Autodesk Inventor part; units mm, degrees
ref_plane "YZ Plane" through (0, 0, 0) normal (1, 0, 0) x (0, 1, 0)
ref_plane "XZ Plane" through (0, 0, 0) normal (0, 1, 0) x (-1, 0, 0)
ref_plane "XY Plane" through (0, 0, 0) normal (0, 0, 1) x (1, 0, 0)
sketch "Sketch1" plane through (0, 0, 0) normal (0, 0, 1) x (1, 0, 0)
  circle A0 centre (0, 0) radius 45
  line L0 (0, 0) -> (0, -60)
  line L1 (0, -60) -> (60, -60)
  line L2 (60, -60) -> (31.8198, -31.8198)
  line L3 (0, -60) -> (-60, -60)
  line L4 (-60, -60) -> (-31.8198, -31.8198)
  line L5 (29.6985, -33.9411) -> (52.7574, -57)
  line L6 (52.7574, -57) -> (0, -57)
  line L7 (-29.6985, -33.9411) -> (-52.7574, -57)
  line L8 (-52.7574, -57) -> (0, -57)
  circle A1 centre (0, 0) radius 49.5
  point P0 (0, -45)
  point P1 (32.8161, -37.0588)
  point P2 (-32.8161, -37.0588)
  dimension "d0" = 90
  dimension "d1" = 60
  dimension "d2" = 60
  dimension "d3" = 45
  dimension "d18" = 3
  dimension "d19" = 3
  dimension "d20" = 4.5
extrude "Extrusion1" add sketch "Sketch1" along normal blind 15 contours A0 L0 A1 L4 | L2 A1 L0 A0 | A1 L7 L8 L0 L3 L4 | L2 L1 L0 L6 L5 A1
sketch "Sketch6" plane through (-60, -60, 0) normal (0, -1, 0) x (1, 0, 0)
  circle A0 centre (60, 7.5) radius 3.5
  line L0 (0, 15) -> (120, 15)
  point P0 (60, 0)
  dimension "d27" = 7
  dimension "d28" = 7.5
extrude "Extrusion6" cut sketch "Sketch6" against normal blind 3
sketch "Sketch7" plane through (-60, -60, 0) normal (0, -1, 0) x (1, 0, 0)
  circle A0 centre (60, 7.5) radius 3.5
  circle A1 centre (60, 7.5) radius 1.25
  point P0 (60, 0)
  dimension "d31" = 2.5
extrude "Extrusion7" cut sketch "Sketch7" against normal blind 21.25 contours A1
chamfer "Chamfer1" distance 2 angle 45 1 edges at (-1.25, -49.4842, 7.5043)
fillet "Fillet1" radius 2 8 edges at (-52.7574, -57, 7.5) (-32.8161, -37.0588, 7.5) (32.8161, -37.0588, 7.5) (52.7574, -57, 7.5) (60, -60, 7.5) (-60, -60, 7.5) (-31.8198, -31.8198, 7.5) (31.8198, -31.8198, 7.5)
properties part number "Horizontal Base_3DPrint"
Geometry: final body of the model. Coordinates: model frame, mm. A direction names the side the tool comes from. Coordinates: 2 decimals unless noted, no trailing zeros. Order: outer loops, then holes, each group sorted by start corner. A loop starts at its lowest first (then second) coordinate and runs counter-clockwise, first axis right, second up. Notation, with made-up numbers: M 53,35.25 L 100,35.25 A12 ccw 100,42.25 Z; hole C -18.75,88 d7. An arc over 180 degrees is marked long. Answer in a Markdown table with one row per item. Add a question column.
Q1. Line query: L1, parallel to Z at x = 0, y = -45.7; L2, parallel to Z at x = 0, y = -58.7; L3, parallel to X at y = -39.5, z = 9.5. Output: solid intervals per line, ascending.
Q2. Reachability of faces 1 (the flat face through (-41.63, -45.87, 7.4)), 2 (the cylindrical face through (31.85, -32.62, 7.6)) from +Z, -Z, +X, -X, +Y, -Y: full face, straight path, thin tool, end or side. Return the list, or none.
Q3. Section query B-B on x = 14.5. Return the cut outline in (y, z), and give its area (3 significant figures).
Q4. Section query C-C on y = -43. Return the cut outline in (x, z).
Q5. Section query D-D on x = 0. Count the separate pieces of the cut face and the enclosed holes in it, and give its area (4 significant figures).
Q6. Section query A-A on z = 12.75. Return the cut outline in (x, y).
Q7. Contact query for flat-ended pins moving along their axis: P1, Ø1, axis at y = -49, z = 8.5, coming from the +X side; P2, Ø8, axis at x = 0, z = 7.5, coming from the +Y side; P3, Ø1.5, axis at y = -45, z = 2.5, coming from the -X side. Output: stop coordinate, or through.
Q8. Mould query, pull axis X, two halves, no side actions, for faces 3 (the flat face through (0, -49, 15)), 4 (the cylindrical face through (-57.032, -58.735, 7.605)), 5 (the cylindrical face through (-0.759, -58.521, 4.083)), 6 (the flat face through (45, -45, 7)). Classes: released by +X, released by -X, zero draft, split by the parting line, or undercut.
Completed:
| question | item | result |
|---|---|---|
| 1 | L1 | z = 0 to 6.25, 8.75 to 15 |
| 1 | L2 | z = 0 to 4, 11 to 15 |
| 1 | L3 | x = -39.5 to -35.26, -29.83 to -21.56, 21.56 to 29.83, 35.26 to 39.5 |
| 2 | face 1 | +Z, -Z |
| 2 | face 2 | +Z, -Z, +Y |
| 3 | outline | M -60,0 L -57,0 L -57,15 L -60,15 Z; M -47.33,0 L -42.6,0 L -42.6,15 L -47.33,15 Z |
| 3 | area | 116 mm2 |
| 4 | outline | M -43,0 L -38.76,0 L -38.76,15 L -43,15 Z; M -24.52,0 L -13.27,0 L -13.27,15 L -24.52,15 Z; M 13.27,0 L 24.52,0 L 24.52,15 L 13.27,15 Z; M 38.76,0 L 43,0 L 43,15 L 38.76,15 Z |
| 5 | separate pieces | 4 |
| 5 | enclosed holes | 0 |
| 5 | area | 76.25 mm2 |
| 6 | outline | M -56.59,-56.59 A2 ccw -55.17,-60 L 55.17,-60 A2 ccw 56.59,-56.59 L 33.2,-33.2 A2 ccw 30.44,-33.15 A45 cw -30.44,-33.15 A2 ccw -33.2,-33.2 Z; hole M -49.34,-53.59 A2 ccw -47.93,-57 L 47.93,-57 A2 ccw 49.34,-53.59 L 34.12,-38.37 A2 ccw 31.44,-38.23 A49.5 cw -31.44,-38.23 A2 ccw -34.12,-38.37 Z |
| 7 | P1 | stops at x = 49.5 |
| 7 | P2 | stops at y = -44.82 |
| 7 | P3 | stops at x = -45.75 |
| 8 | face 3 | zero draft |
| 8 | face 4 | released by -X |
| 8 | face 5 | undercut |
| 8 | face 6 | released by +X |
